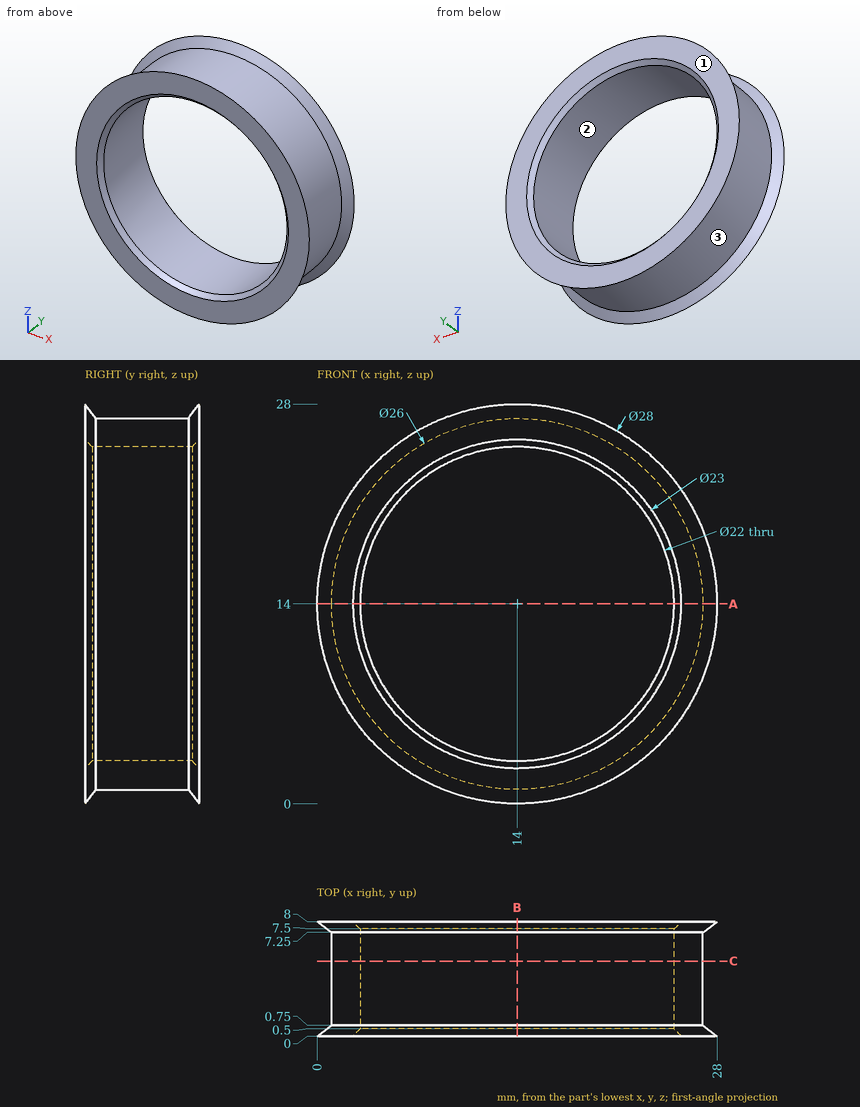
Could you check a few things on this drawing? It's one solid part, dimensions in mm from its lowest x, y, z. Coordinates: 2 decimals unless noted, no trailing zeros. Order: outer loops, then holes, each group sorted by start corner. A loop starts at its lowest first (then second) coordinate and runs counter-clockwise, first axis right, second up. Notation, with made-up numbers: (-33, -8) - (23, -8) arc R27 cw to (23, 25) - close; hole circle Ø7 at (-17.5, 86). An arc over 180 degrees is marked (long way). One line per question, with ' | ' between items.
(1) If we mould it in two halves opening along Z, with no side actions, what happens to the marked faces 1, 2 and 3? For each: pulls with the +Z half, pulls with the -Z half, needs draft (parallel to the pull), parting line crosses it, or undercut.
Report:
face 1: needs draft | face 2: undercut | face 3: parting line crosses it
(2) Suppose I cut it at C-C on y = 5.25. List the corners of the cut face in (x, z) for me, and give its area (3 significant figures).
Report:
outline: circle Ø26 at (14, 14); hole circle Ø22 at (14, 14) | area: 151 mm2
(3) Suppose I cut it at A-A on z = 14. List the corners of the cut face in (x, y) for me.
Report:
outline: (0, 0) - (2.5, 0) - (3, 0.5) - (3, 7.5) - (2.5, 8) - (0, 8) - (1, 7.25) - (1, 0.75) - close; (25, 0.5) - (25.5, 0) - (28, 0) - (27, 0.75) - (27, 7.25) - (28, 8) - (25.5, 8) - (25, 7.5) - close
(4) If I drill on L1, parallel to Z at x = 14, y = 3; L2, parallel to Z at x = 19, y = 4.25; L3, parallel to X at y = 4.25, z = 4.75, over which ranges is the centre line in solid material (lowest first)?
Report:
L1: z = 1 to 3, 25 to 27 | L2: z = 2 to 4.2, 23.8 to 26 | L3: x = 4.87 to 8.05, 19.95 to 23.13
(5) Will these pins go through, and if not, where does the flat tip stop? pin 1 (3 mm diameter, centred on y = 3, z = 18, fed in from +X); pin 2 (2 mm diameter, centred on x = 4.5, z = 18, fed in from +Y); pin 3 (2 mm diameter, centred on x = 9.5, y = 5, fed in from -Z).
Report:
pin 1: stops at x = 26.76 | pin 2: stops at y = 7.81 | pin 3: stops at z = 1.48
(6) Suppose I cut it at B-B on x = 14. List the corners of the cut face in (y, z) for me, and give its area (3 significant figures).
Report:
outline: (0, 0) - (0.75, 1) - (7.25, 1) - (8, 0) - (8, 2.5) - (7.5, 3) - (0.5, 3) - (0, 2.5) - close; (0, 25.5) - (0.5, 25) - (7.5, 25) - (8, 25.5) - (8, 28) - (7.25, 27) - (0.75, 27) - (0, 28) - close | area: 33.0 mm2
